Read the model definition and answer for the solid it produces. Units are mm, in the model's axes. Face numbers are marked on the shaded views. A direction names the side the tool comes from. Give positions to 0.01 mm unless a question says otherwise; leave off trailing zeros. Order: outer loops, then holes, each group sorted by start corner. A loop starts at its lowest first (then second) coordinate and runs counter-clockwise, first axis right, second up. Notation, with made-up numbers: (25, 29.25) -> (39, 29.25) arc R31 cw to (39, 65.25) -> close; hole circle Ø4 at (0, -2). An arc over 180 degrees is marked (long way). Answer as CSV lines item,"result". Start each with the question number.
1) Find section C-C (y = 12). Determine the outline of the cut face in (x, z).
2) Straight lines are drawn through the part: L1, parallel to X at y = 0.3, z = 40; L2, parallel to Y at x = 12.5, z = 1.7; L3, parallel to Z at x = 3.25, y = 9.25. For each, find the intervals that lie inside material, in ascending order. Write a range as from..to.
3) Flat-ended cylindrical pins translate along their axes: pin 1 Ø8 at (x, y) = (18.5, 9) entering from +Z; pin 2 Ø10 at (x, z) = (22, 35.5) entering from +Y; pin 3 Ø6 at (x, y) = (10.5, 13.5) entering from -Z; pin 4 Ø6.5 at (x, z) = (12.5, 40) entering from +Y. Find the tip coordinate at first contact, or state that the pin passes through.
4) The mould has two halves that part along Z. Classify the marked faces 3, 4 and 5: +Z half, -Z half, draft (parallel to the pull), parting line (faces both ways), or undercut.
5) Find section A-A (z = 40). Determine the outline of the cut face in (x, y), and give its area (3 significant figures).
6) Find section D-D (x = 5.25). Determine the outline of the cut face in (y, z).
7) Find section B-B (x = 12.5). Determine the outline of the cut face in (y, z), and give its area (3 significant figures).
8) For the marked faces 1 and 2, determine the directions among +Z, -Z, +X, -X, +Y, -Y from which every point of the face is accessible in a straight line to the end or side of a thin tool.
```python
from build123d import *

# Parameters (mm, degrees)
T_LE_DE_BASE_PLI_E1_DEPTH = 25
D_GAGEMENT_M81_D          = 9


# Sheet-metal steps are written as plain solids
with BuildPart() as part:
    # Esquisse1 → Tôle de base pliée1 (new body)
    with BuildSketch(Plane(origin=(0, 0, 0), x_dir=(0, 0, -1), z_dir=(1, 0, 0))):
        with BuildLine():
            Line((0, 20), (0, 4))
            ThreePointArc((0, 4), (-1.171572875, 1.171572875), (-4, 0))
            Line((-4, 0), (-48, 0))
            Line((-48, 0), (-48, 3))
            Line((-48, 3), (-4, 3))
            ThreePointArc((-4, 3), (-3.292893219, 3.292893219), (-3, 4))
            Line((-3, 4), (-3, 20))
            Line((-3, 20), (0, 20))
        make_face()
    extrude(amount=T_LE_DE_BASE_PLI_E1_DEPTH)

    # Esquisse3 → Fraisage pour vis à tête fraisée M51 (revolve, cut)
    with BuildSketch(Plane(origin=(12.5, 3, 40), x_dir=(0, 0, 1), z_dir=(1, 0, 0))):
        Polygon((0, 0), (0, 3), (2.75, 3), (2.75, 2.45), (5.2, 0), align=None)
    revolve(axis=Axis((12.5, 9.35, 40), (0, -1, 0)), mode=Mode.SUBTRACT)

    # Dégagement M81 (through all)
    with Locations(Plane.XY.offset(3)):
        with Locations((12.5, 12)):
            Hole(D_GAGEMENT_M81_D / 2)


solid = part.part
```
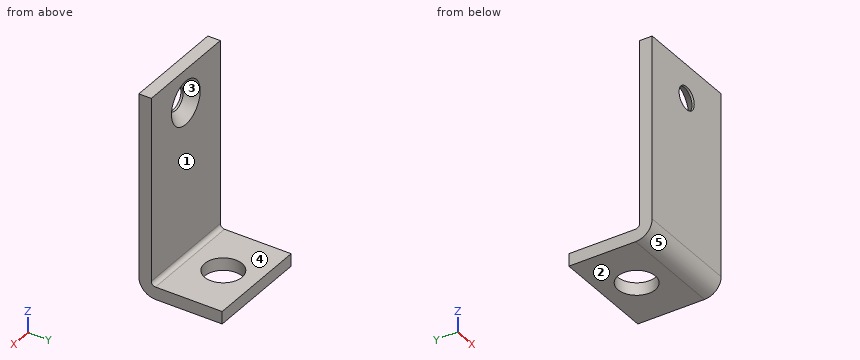
Findings below:
1,outline,"(0, 0) -> (8, 0) -> (8, 3) -> (0, 3) -> close; (17, 0) -> (25, 0) -> (25, 3) -> (17, 3) -> close"
2,L1,"0..9.75, 15.25..25"
2,L2,"0.73..7.5, 16.5..20"
2,L3,"0..3"
3,pin 1,"z = 3"
3,pin 2,"y = 3"
3,pin 3,"z = 0"
3,pin 4,"y = 1.05"
4,face 3,"undercut"
4,face 4,"+Z half"
4,face 5,"-Z half"
5,outline,"(0, 0) -> (9.75, 0) -> (9.75, 0.55) -> (7.3, 3) -> (0, 3) -> close; (15.25, 0) -> (25, 0) -> (25, 3) -> (17.7, 3) -> (15.25, 0.55) -> close"
5,area,"52.5 mm²"
6,outline,"(0, 4) arc R4 ccw to (4, 0) -> (20, 0) -> (20, 3) -> (4, 3) arc R1 cw to (3, 4) -> (3, 48) -> (0, 48) -> close"
7,outline,"(0, 4) arc R4 ccw to (4, 0) -> (7.5, 0) -> (7.5, 3) -> (4, 3) arc R1 cw to (3, 4) -> (3, 34.8) -> (0.55, 37.25) -> (0, 37.25) -> close; (0, 42.75) -> (0.55, 42.75) -> (3, 45.2) -> (3, 48) -> (0, 48) -> close; (16.5, 0) -> (20, 0) -> (20, 3) -> (16.5, 3) -> close"
7,area,"142 mm²"
8,face 1,"+Z, +X, -X, +Y"
8,face 2,"-Z, +X, -X, +Y, -Y"
